Could you check a few things on this model? Use its own coordinates, in mm. Face numbers are marked on the shaded views. A direction names the side the tool comes from. Give positions to 0.01 mm unless a question says otherwise; leave off trailing zeros. Order: outer loops, then holes, each group sorted by start corner. A loop starts at its lowest first (then second) coordinate and runs counter-clockwise, first axis right, second up. Notation, with made-up numbers: M -22.75,87.25 L 31.25,87.25 A8 ccw 31.25,92.25 Z; hole C 87.25,83 d5. An arc over 180 degrees is marked long. Answer in a Markdown table with one row per item. Add a question column.
```python
from build123d import *

# Parameters (mm, degrees)
SKETCH2_R          = 2.33256351
HEX_DIE_DEPTH      = 11
SKETCH5_R          = 1.003913097
CUT_EXTRUDE1_DEPTH = 6


with BuildPart() as part:
    # BodySke → Base-Revolve (revolve)
    with BuildSketch(Plane.XY, mode=Mode.PRIVATE) as base_revolve_sk:
        Polygon((11, 1.25), (11, 2.309468822), (0.178671908, 2.309468822), (0, 2), (0, 0), (17, 0), (17, 1.25), align=None)
    revolve(base_revolve_sk.sketch.rotate(Axis((-25.4, 0, 0), (1, 0, 0)), 90), axis=Axis((-25.4, 0, 0), (1, 0, 0)))

    # Sketch2 → Hex-Die (cut)
    with BuildSketch(Plane(origin=(0, 0, 0), x_dir=(0, 0, -1), z_dir=(1, 0, 0))):
        Circle(SKETCH2_R)
        Polygon((-2, 1.154700543), (0, 2.309401087), (2, 1.154700543), (2, -1.154700543), (0, -2.309401087), (-2, -1.154700543), align=None, mode=Mode.SUBTRACT)
    extrude(amount=HEX_DIE_DEPTH, mode=Mode.SUBTRACT)

    # Sketch5 → Cut-Extrude1 (cut)
    with BuildSketch(Plane.ZY):
        Circle(SKETCH5_R)
    extrude(amount=-CUT_EXTRUDE1_DEPTH, mode=Mode.SUBTRACT)


solid = part.part
```
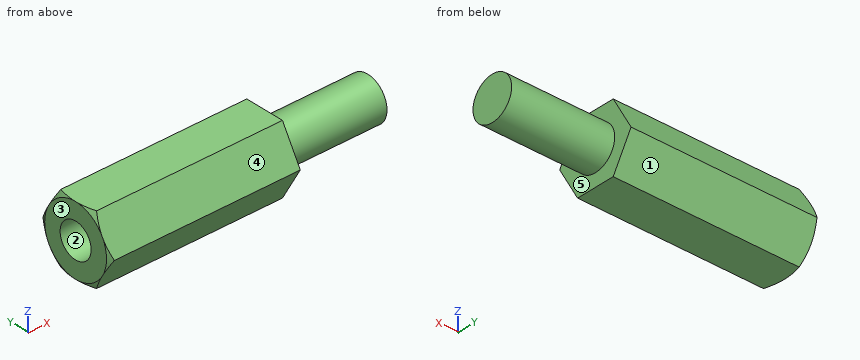
1. Suppose I cut it at A-A on x = 9. List the corners of the cut face in (y, z) for me.
2. Thinking about a two-plate mould opening in Y: for the marked faces 1, 2 and 3, which applies, pulls with the +Y half, pulls with the -Y half, needs draft (parallel to the pull), parting line crosses it, or undercut?
3. Suppose I cut it at B-B on x = 15.25. List the corners of the cut face in (y, z) for me.
4. Will these pins go through, and if not, where does the flat tip stop? P1, Ø2, axis at x = 14.5, z = 1.5, coming from the -Y side; P2, Ø1, axis at x = 6.5, z = -1, coming from the +Y side; P3, Ø1.5, axis at x = 3.5, y = 1.5, coming from the -Z side.
5. For the marked faces 4 and 5, which set-ups out of +Z, -Z, +X, -X, +Y, -Y let a thin tool reach every point of the face, with its end or its side?
6. If I drill on line 1 along X through (y, z) = (0, 0.6); line 2 along X through (y, z) = (-0.2, 1.35); line 3 along Z through (x, y) = (15.5, -0.05), over which ranges is the centre line in solid material (lowest first)? Write a range as [from, to].
Findings below:
| question | item | result |
|---|---|---|
| 1 | outline | M -2.31,0 L -1.15,-2 L 1.15,-2 L 2.31,0 L 1.15,2 L -1.15,2 Z |
| 2 | face 1 | pulls with the +Y half |
| 2 | face 2 | undercut |
| 2 | face 3 | needs draft |
| 3 | outline | C 0,0 d2.5 |
| 4 | P1 | y = -1.15 |
| 4 | P2 | y = 2.02 |
| 4 | P3 | z = -2 |
| 5 | face 4 | +Z, +X, -X, -Y |
| 5 | face 5 | +X |
| 6 | line 1 | [6, 17] |
| 6 | line 2 | [0, 11] |
| 6 | line 3 | [-1.25, 1.25] |
